Here's how the part is built. I have some questions about the finished solid (model axes, mm). A direction names the side the tool comes from. Round coordinates to 2 decimals unless told otherwise and drop trailing zeros. Order: outer loops, then holes, each group sorted by start corner. A loop starts at its lowest first (then second) coordinate and runs counter-clockwise, first axis right, second up.
Autodesk Inventor part; units mm, degrees
ref_plane "YZ Plane" through (0, 0, 0) normal (1, 0, 0) x (0, 1, 0)
ref_plane "XZ Plane" through (0, 0, 0) normal (0, 1, 0) x (-1, 0, 0)
ref_plane "XY Plane" through (0, 0, 0) normal (0, 0, 1) x (1, 0, 0)
sketch "Sketch1" plane through (0, 0, 0) normal (1, 0, 0) x (0, 1, 0)
  line L0 (0, 0) -> (12.7, 0)
  line L1 (12.7, 0) -> (12.7, -25.4)
  line L2 (12.7, -25.4) -> (0, -25.4)
  line L3 (0, -25.4) -> (0, 0)
  dimension "d0" = 12.7
  dimension "d1" = 25.4
extrude "Extrusion1" add sketch "Sketch1" along normal blind 125.6538
sketch "Sketch3" plane through (0, 12.7, 0) normal (0, 1, 0) x (1, 0, 0)
  line L0 (0, 0) -> (125.6538, 0)
  line L1 (0, 25.4) -> (125.6538, 25.4)
  circle A0 centre (11.1125, 12.7) radius 6.35
  circle A1 centre (114.5413, 12.7) radius 6.35
  point P0 (36.5125, 12.7)
  point P1 (60.5125, 12.7)
  dimension "d13" = 25.4
  dimension "d14" = 12.7
  dimension "d16" = 24
  dimension "d36" = 25.4
hole "Hole1" at (36.5125, 12.7, -12.7) at (60.5125, 12.7, -12.7) direction (0, -1, 0) diameter 3 end through all
sketch "Sketch5" plane through (0, 12.7, 0) normal (0, 1, 0) x (1, 0, 0)
  line L0 (0, 0) -> (125.6538, 0)
  line L1 (0, 25.4) -> (125.6538, 25.4)
  circle A0 centre (114.5413, 12.7) radius 6.35
  point P0 (95.4913, 12.7)
  dimension "d26" = 12.7
  dimension "d27" = 25.4
  dimension "d28" = 19.05
hole "Hole2" at (95.4913, 12.7, -12.7) direction (0, -1, 0) diameter 3.302 end through all
sketch "Sketch12" plane through (0, 12.7, 0) normal (0, 1, 0) x (1, 0, 0)
  circle A0 centre (95.4913, 12.7) radius 1.651
  circle A1 centre (36.5125, 12.7) radius 1.5
  circle A2 centre (60.5125, 12.7) radius 1.5
  line L0 (0, 0) -> (0, 25.4)
  line L1 (0, 0) -> (125.6538, 0)
  line L2 (125.6538, 25.4) -> (125.6538, 0)
  line L3 (0, 25.4) -> (125.6538, 25.4)
  point P0 (0, 0)
  point P1 (82.7913, 12.7)
  dimension "d77" = 12.7
  dimension "d78" = 12.7
  dimension "d79" = 12.7
hole "Hole5" at (82.7913, 12.7, -12.7) direction (0, -1, 0) diameter 3.302 end through all
sketch "Sketch14" plane through (0, 12.7, 0) normal (0, 1, 0) x (1, 0, 0)
  circle A0 centre (82.7913, 12.7) radius 1.651
  circle A1 centre (95.4913, 12.7) radius 1.651
  circle A2 centre (36.5125, 12.7) radius 1.5
  circle A3 centre (60.5125, 12.7) radius 1.5
  line L0 (0, 0) -> (0, 25.4)
  line L1 (0, 0) -> (125.6538, 0)
  line L2 (125.6538, 25.4) -> (125.6538, 0)
  line L3 (0, 25.4) -> (125.6538, 25.4)
  point P0 (0, 0)
  point P1 (11.1125, 12.7)
hole "Hole7" at (11.1125, 12.7, -12.7) direction (0, -1, 0) diameter 7.62 end through all
sketch "Sketch15" plane through (0, 12.7, 0) normal (0, 1, 0) x (1, 0, 0)
  circle A0 centre (11.1125, 12.7) radius 3.81
  circle A1 centre (82.7913, 12.7) radius 1.651
  circle A2 centre (95.4913, 12.7) radius 1.651
  circle A3 centre (36.5125, 12.7) radius 1.5
  circle A4 centre (60.5125, 12.7) radius 1.5
  line L0 (0, 0) -> (0, 25.4)
  line L1 (0, 0) -> (125.6538, 0)
  line L2 (125.6538, 25.4) -> (125.6538, 0)
  line L3 (0, 25.4) -> (125.6538, 25.4)
  circle A5 centre (114.5413, 12.7) radius 4.7625
  point P0 (0, 0)
hole "Hole8" at (114.5413, 12.7, -12.7) direction (0, -1, 0) diameter 9.525 end through all
sketch "Sketch16" plane through (0, 12.7, 0) normal (0, 1, 0) x (1, 0, 0)
  circle A0 centre (114.5413, 12.7) radius 4.7625
  circle A1 centre (11.1125, 12.7) radius 3.81
  circle A2 centre (82.7913, 12.7) radius 1.651
  circle A3 centre (95.4913, 12.7) radius 1.651
  circle A4 centre (36.5125, 12.7) radius 1.5
  circle A5 centre (60.5125, 12.7) radius 1.5
  line L0 (0, 0) -> (0, 25.4)
  line L1 (0, 0) -> (125.6538, 0)
  line L2 (125.6538, 25.4) -> (125.6538, 0)
  line L3 (0, 25.4) -> (125.6538, 25.4)
  line L4 (0, 0) -> (125.6538, 0)
  line L5 (0, 0) -> (25.4, 0)
  line L6 (25.4, 0) -> (25.4, 25.4)
  line L7 (25.4, 25.4) -> (0, 25.4)
  line L8 (0, 25.4) -> (0, 0)
  dimension "d110" = 25.4
extrude "Extrusion7" cut sketch "Sketch16" against normal blind 6.35 contours L0 L3 L6 L1
properties part number "L17_TSI_010"
1. I'm going to push flat-ended pins straight in: P1, Ø12.5, axis at x = 7, z = -11.5, coming from the +Y side; P2, Ø1.9, axis at y = 10.5, z = -8.5, coming from the -X side. Where does each tip first touch, or does it pass through?
Evaluation:
P1: stops at y = 6.35
P2: stops at x = 25.4
2. I need wall thicknesses on probe 1 along Z at (x, y) = (118, 7.5); probe 2 along Y at (x, z) = (21, -9); probe 3 along Z at (x, y) = (116.5, 5.75). Which ranges of each line are inside material? Lowest first, please.
Evaluation:
probe 1: z = -25.4 to -15.97, -9.43 to 0
probe 2: y = 0 to 6.35
probe 3: z = -25.4 to -17.04, -8.36 to 0
3. If we section it at A-A, the plane z = -12.7: State how many separate pieces and enclosed holes the cut face has, and give its area (3 significant figures).
Evaluation:
separate pieces: 7
enclosed holes: 0
area: 1,110 mm2
4. If we section it at D-D, the plane x = 20.5: Write out the boundary of the cut face in (y, z).
Evaluation:
outline: (0, -25.4) - (6.35, -25.4) - (6.35, 0) - (0, 0) - close
5. If we section it at B-B, the plane y = 11: Write out the boundary of the cut face in (x, z) (1 decimal).
Evaluation:
outline: (25.4, -25.4) - (125.7, -25.4) - (125.7, 0) - (25.4, 0) - close; hole circle Ø3 at (36.5, -12.7); hole circle Ø3 at (60.5, -12.7); hole circle Ø3.3 at (82.8, -12.7); hole circle Ø3.3 at (95.5, -12.7); hole circle Ø9.5 at (114.5, -12.7)
6. On a 3-axis mill with a long thin cutter (end or side, diameter ignored), from which of +Z, -Z, +X, -X, +Y, -Y can I reach the whole of each face in a straight line? I mean faces 4 (the cylindrical face through (81.154, 6.261, -12.915)), 5 (the flat face through (15.3, 6.35, -12.9)). Say none if no direction works.
Evaluation:
face 4: +Y, -Y
face 5: +Z, -Z, -X, +Y
7. If we mould it in two halves opening along X, with no side actions, what happens to faces 1 (the flat face through (125.654, 6, -13)), 2 (the flat face through (62, 6, 0)), 3 (the cylindrical face through (8.54, 3.13, -15.51))? For each: released by +X, released by -X, zero draft, split by the parting line, or undercut.
Evaluation:
face 1: released by +X
face 2: zero draft
face 3: undercut
8. If we section it at C-C, the plane y = 3.25: Write out the boundary of the cut face in (x, z) (1 decimal), and give its area (3 significant figures).
Evaluation:
outline: (0, -25.4) - (125.7, -25.4) - (125.7, 0) - (0, 0) - close; hole circle Ø7.6 at (11.1, -12.7); hole circle Ø3 at (36.5, -12.7); hole circle Ø3 at (60.5, -12.7); hole circle Ø3.3 at (82.8, -12.7); hole circle Ø3.3 at (95.5, -12.7); hole circle Ø9.5 at (114.5, -12.7)
area: 3,040 mm2
